from build123d import *

# Parameters (mm, degrees)
F1_DEPTH = 34.544
F2_R     = 2.54
F3_DEPTH = 34.545


with BuildPart() as f1:
    # F0 (on Top) → F1 (new body)
    with BuildSketch(Plane.XY):
        Polygon((5.259377, 1.2315), (0.45401, 5.382519), (-4.978783, 2.095079), (-3.531067, -4.087689), (2.796463, -4.62141), align=None)
    extrude(amount=F1_DEPTH)

    # F2 (on face) → F3 (cut, through all)
    with BuildSketch(Plane.XY.offset(34.544)):
        Circle(F2_R)
    extrude(amount=-F3_DEPTH, mode=Mode.SUBTRACT)


solid = f1.part
Verification items for the finished model (mm, model axes). Coordinates: 2 decimals unless noted, no trailing zeros. Write each loop counter-clockwise with the first axis right and the second up, starting at its lowest first coordinate (ties: lowest second). Pieces come first, ordered by that corner, then holes. Notation, with made-up numbers: M 45,66 L 93,66 A27 cw 93,102 Z; hole C 41,27.5 d2. An arc over 180 degrees is marked long. Use a Markdown table: item, result.
Q1. Sectioned sample at B-B, the plane y = -0.75. Record the boundary of the cut face in (x, z).
Reply:
| item | result |
|---|---|
| outline | M -4.31,0 L -2.43,0 L -2.43,34.54 L -4.31,34.54 Z; M 2.43,0 L 4.43,0 L 4.43,34.54 L 2.43,34.54 Z |
Q2. Sectioned sample at A-A, the plane z = 24. Record the boundary of the cut face in (x, y), plus the area to 3 significant figures.
Reply:
| item | result |
|---|---|
| outline | M -4.98,2.1 L -3.53,-4.09 L 2.8,-4.62 L 5.26,1.23 L 0.45,5.38 Z; hole C 0,0 d5.08 |
| area | 49.1 mm² |
Q3. Go/stop test with flat-tipped pins: P1, Ø4, axis at x = -1, z = 19, coming from the -Y side; P2, Ø3, axis at y = 0.5, z = 4, coming from the -X side. Record where each tip stops, or that it passes through.
Reply:
| item | result |
|---|---|
| P1 | stops at y = -4.47 |
| P2 | stops at x = -4.96 |
Q4. Draft check along Y on faces 1 (the face through (-2, -2, 34.544)), 2 (the face through (-0.33, 2.52, 17.51)), 3 (the face through (-4.265, -0.953, 17.03)), 4 (the face through (2.89, 3.28, 17.03)). Enter one of: +Y half, -Y half, draft (parallel to the pull), parting line (faces both ways), or undercut.
Reply:
| item | result |
|---|---|
| face 1 | draft |
| face 2 | undercut |
| face 3 | -Y half |
| face 4 | +Y half |
Q5. Sectioned sample at D-D, the plane y = -3.5. Record the boundary of the cut face in (x, z), plus the area to 3 significant figures.
Reply:
| item | result |
|---|---|
| outline | M -3.67,0 L 3.27,0 L 3.27,34.54 L -3.67,34.54 Z |
| area | 240 mm² |
Q6. Sectioned sample at C-C, the plane x = 1. Record the boundary of the cut face in (y, z), plus the area to 3 significant figures.
Reply:
| item | result |
|---|---|
| outline | M -4.47,0 L -2.33,0 L -2.33,34.54 L -4.47,34.54 Z; M 2.33,0 L 4.91,0 L 4.91,34.54 L 2.33,34.54 Z |
| area | 163 mm² |
Q7. Thickness scan on line 1 (Y direction, x = 1.75, z = 9); line 2 (Y direction, x = 0, z = 9); line 3 (X direction, y = 1.5, z = 33.5). Record the ranges inside material, lowest first.
Reply:
| item | result |
|---|---|
| line 1 | y = -4.53 to -1.84, 1.84 to 4.26 |
| line 2 | y = -4.39 to -2.54, 2.54 to 5.11 |
| line 3 | x = -4.84 to -2.05, 2.05 to 4.95 |
